Check sheet for the modelled part. Datum: model origin and axes. Units: mm. A direction names the side the tool comes from. Give positions to 0.01 mm unless a question says otherwise; leave off trailing zeros. Order: outer loops, then holes, each group sorted by start corner. A loop starts at its lowest first (then second) coordinate and runs counter-clockwise, first axis right, second up. Notation, with made-up numbers: M -3.75,85.25 L 11.25,85.25 A11 cw 11.25,94.25 Z; hole C 34,89 d6. An arc over 180 degrees is marked long. Answer in a Markdown table with one row per item. Add a question column.
from build123d import *

# Parameters (mm, degrees)
F1_DEPTH = 355.6
F3_DEPTH = 3.175
F6_DEPTH = 3.175
F8_D     = 9.525
F8_DEPTH = 5.08
F8_TIP   = 2.8615986981
F9_R     = 1.27


with BuildPart() as f1:
    # F0 (on Right) → F1 (new body)
    with BuildSketch(Plane.YZ):
        Polygon((118.5154446509, -25.4), (-110.0845239475, 0), (-110.0845239475, -3.175), (121.6904760525, -28.9277813153), (121.6904760525, 44.8288065905), (118.5154760525, 44.8288080101), align=None)
        Polygon((-110.0845239475, -3.175), (-110.0845239475, 0), (-113.2595239475, 0), (-113.2595239475, -38.1), (-110.0845239475, -38.1), align=None)
    extrude(amount=-F1_DEPTH)

    # F2 (on Right) → F3 (join)
    with BuildSketch(Plane.YZ):
        Polygon((-113.2595239475, 44.8288080101), (-113.2595239475, 0), (-110.0845239475, 0), (118.5154446509, -25.4), (118.5154760525, 44.8288080101), align=None)
    extrude(amount=-F3_DEPTH)

    # F5 (on offset) → F6 (join)
    with BuildSketch(Plane.YZ.offset(-355.6)):
        Polygon((118.5154760525, 44.8288080101), (-113.2595239475, 44.8288080101), (-113.2595239475, 0), (-110.0845239475, 0), (118.5154446509, -25.4), align=None)
    extrude(amount=F6_DEPTH)

    # F8
    with Locations(Plane.XZ.offset(113.2595239475)):
        with Locations((-236.982, -19.05), (-118.618, -19.05)):
            Hole(F8_D / 2, depth=F8_DEPTH)
            with Locations((0, 0, -(F8_DEPTH + F8_TIP / 2))):  # 118° drill point
                Cone(0, F8_D / 2, F8_TIP, mode=Mode.SUBTRACT)

    # F9
    f9_edges = [f1.edges().sort_by_distance(p)[0] for p in [
        (-352.425, 118.51546, 9.714404),
        (-3.175, 118.51546, 9.714404),
        (-355.6, 2.627976, 44.828808),
        (0, 2.627976, 44.828808),
        (-177.8, 121.690476, 44.828807),
    ]]
    fillet(f9_edges, radius=F9_R)


solid = f1.part
Q1. Tool access check on faces 1 (the flat face through (0, 3, 12)), 2 (the flat face through (-175, -110.085, -21)), 3 (the flat face through (-352.425, 0, 18)), 4 (the cylindrical face through (-232.224, -111.65, -18.841)), 5 (the flat face through (-355.6, 3, 12)). Record the directions out of +Z, -Z, +X, -X, +Y, -Y that give a thin tool (end or side, any length) a straight path to the whole face; none if there is none.
Q2. Cross-section at C-C (z = -19.05). State how many separate pieces and enclosed holes the cut face has, and give its area (3 significant figures).
Q3. Draft check along Y on faces 6 (the flat face through (-180, -113.26, -24)), 7 (the flat face through (-175, 121.69, 7)), 8 (the flat face through (-175.31, 4.18, -15.87)). Enter one of: pulls with the +Y half, pulls with the -Y half, needs draft (parallel to the pull), parting line crosses it, or undercut.
Q4. Thickness scan on probe 1 along X at (y, z) = (32.5, -8.5) (3 decimals); probe 2 along Y at (x, z) = (-128.5, 4); probe 3 along Y at (x, z) = (-144.5, -31). Record the ranges inside material, lowest first.
Q5. Cross-section at A-A (x = -322). Record the boundary of the cut face in (y, z) (3 decimals), and give its area (3 significant figures).
Q6. Cross-section at B-B (y = 5). Record the boundary of the cut face in (x, z) (3 decimals), and give its area (3 significant figures).
Q7. Go/stop test with flat-tipped pins: pin 1 (3 mm diameter, centred on x = -279, y = 9, fed in from +Z); pin 2 (10 mm diameter, centred on x = -164, z = 2.5, fed in from -Y); pin 3 (8 mm diameter, centred on x = -245, y = 97.5, fed in from +Z); pin 4 (1 mm diameter, centred on x = -167, y = -111, fed in from +Z). Record where each tip stops, or that it passes through.
Values follow:
| question | item | result |
|---|---|---|
| 1 | face 1 | +Z, -Z, +X, +Y, -Y |
| 1 | face 2 | -Z, +X, -X |
| 1 | face 3 | +Z |
| 1 | face 4 | -Y |
| 1 | face 5 | +Z, -Z, -X, +Y, -Y |
| 2 | separate pieces | 4 |
| 2 | enclosed holes | 1 |
| 2 | area | 12,700 mm² |
| 3 | face 6 | pulls with the -Y half |
| 3 | face 7 | pulls with the +Y half |
| 3 | face 8 | undercut |
| 4 | probe 1 | -355.6 to -352.425, -3.175 to 0 |
| 4 | probe 2 | 118.52 to 121.69 |
| 4 | probe 3 | -113.26 to -110.08 |
| 5 | outline | M -113.26,-38.1 L -110.085,-38.1 L -110.085,-3.175 L 121.69,-28.928 L 121.69,43.559 A1.27 ccw 120.42,44.829 L 118.515,44.829 L 118.515,-25.4 L -110.085,0 L -113.26,0 Z |
| 5 | area | 1,080 mm² |
| 6 | outline | M -355.6,-15.962 L 0,-15.962 L 0,43.559 A1.27 ccw -1.27,44.829 L -3.175,44.829 L -3.175,-12.787 L -352.425,-12.787 L -352.425,44.829 L -354.33,44.829 A1.27 ccw -355.6,43.559 Z |
| 6 | area | 1,490 mm² |
| 7 | pin 1 | z = -13.06 |
| 7 | pin 2 | y = -113.26 |
| 7 | pin 3 | z = -22.62 |
| 7 | pin 4 | z = 0 |
